Autodesk Inventor part; units mm, degrees
ref_plane "YZ Plane" through (0, 0, 0) normal (1, 0, 0) x (0, 1, 0)
ref_plane "XZ Plane" through (0, 0, 0) normal (0, 1, 0) x (-1, 0, 0)
ref_plane "XY Plane" through (0, 0, 0) normal (0, 0, 1) x (1, 0, 0)
sketch "Skizze1" plane through (0, 0, 0) normal (0, 1, 0) x (-1, 0, 0)
  line L0 (102, -1.5) -> (-102, -1.5)
  line L1 (-102, -1.5) -> (-102, 1.5)
  line L2 (-102, 1.5) -> (102, 1.5)
  line L3 (102, 1.5) -> (102, -1.5)
  line L4 (104, -3.5) -> (-104, -3.5)
  line L5 (-104, -3.5) -> (-104, 3.5)
  line L6 (-104, 3.5) -> (104, 3.5)
  line L7 (104, 3.5) -> (104, -3.5)
  line L8 (0, -4.9) -> (0, 4.9)
  line L9 (-145.6, 0) -> (145.6, 0)
  point P0 (0, 0)
  dimension "d0" = 204
  dimension "d2" = 3
  dimension "d3" = 2
  dimension "d4" = 2
extrude "Extrusion1" add sketch "Skizze1" along normal blind 15 contours L3 L9 L7 L4 L8 L0 | L8 L4 L5 L9 L1 L0 | L3 L2 L8 L6 L7 L9 | L9 L5 L6 L8 L2 L1
sketch "Skizze2" plane through (0, 0, 0) normal (0, 1, 0) x (-1, 0, 0)
  line L0 (104, 3.5) -> (-104, 3.5)
  line L1 (104, -3.5) -> (104, 3.5)
  line L2 (-104, -3.5) -> (104, -3.5)
  line L3 (-104, 3.5) -> (-104, -3.5)
  point P0 (0, 0)
extrude "Extrusion2" add sketch "Skizze2" along normal blind 1
draft "Flächenverjüngung1" angle 10 pull direction (0, 1, 0) faces at (34.6667, 5, -3.5) (104, 10, 1.1667) (-34.6667, 5, 3.5) (-104, 10, -1.1667) fixed edges at (0, 15, -3.5) (104, 15, 0) (0, 15, 3.5) (-104, 15, 0)
properties part number "Stroemungsfilter_Fuss"
Design review of the part built by this model. Coordinates are the model's own, in mm. A direction names the side the tool comes from. Give positions to 0.01 mm unless a question says otherwise; leave off trailing zeros. Write each loop counter-clockwise with the first axis right and the second up, starting at its lowest first coordinate (ties: lowest second). Pieces come first, ordered by that corner, then holes. Notation, with made-up numbers: (77.25, 70) -> (96.25, 70) arc R8 cw to (96.25, 74) -> close; hole circle Ø8 at (4, 51.5). An arc over 180 degrees is marked (long way). Answer in a Markdown table with one row per item.
(1) Consider section A-A (x = 78). State the section outline as (y, z) points.
Results:
| item | result |
|---|---|
| outline | (0, -6.14) -> (15, -3.5) -> (15, -1.5) -> (1, -1.5) -> (1, 1.5) -> (15, 1.5) -> (15, 3.5) -> (0, 6.14) -> close |
(2) For faces 1 (the flat face through (-105.34, 7.39, 0.09)), 2 (the flat face through (1, 8, 1.5)), list the 3-axis set-ups (+Z, -Z, +X, -X, +Y, -Y) from which the entire face can be reached by the end or side of a thin tool; tool diameter is ignored.
Results:
| item | result |
|---|---|
| face 1 | +Z, -Z, -X, +Y |
| face 2 | +Y |
(3) Consider section B-B (y = 6.5). State the section outline as (x, z) points, then the cut area to 3 significant figures.
Results:
| item | result |
|---|---|
| outline | (-105.5, -5) -> (105.5, -5) -> (105.5, 5) -> (-105.5, 5) -> close; hole (-102, -1.5) -> (102, -1.5) -> (102, 1.5) -> (-102, 1.5) -> close |
| area | 1,500 mm2 |
(4) To check wall thickness, follow probe 1 along Z at (x, y) = (92, 11); probe 2 along Z at (x, y) = (32.5, 12.75); probe 3 along X at (y, z) = (9.25, 0.5). State the ranges of each line that lie inside material, in increasing order.
Results:
| item | result |
|---|---|
| probe 1 | -4.21 to -1.5, 1.5 to 4.21 |
| probe 2 | -3.9 to -1.5, 1.5 to 3.9 |
| probe 3 | -105.01 to -102, 102 to 105.01 |
(5) Mouldability with a two-part tool opening along X and no side actions: class faces 3 (the flat face through (-1.49, 7.4, -4.84)), 4 (the flat face through (-1, 8, -1.5)), 5 (the flat face through (105.34, 7.4, -0.09)) as +X half, -X half, draft (parallel to the pull), parting line (faces both ways), or undercut.
Results:
| item | result |
|---|---|
| face 3 | draft |
| face 4 | undercut |
| face 5 | +X half |
(6) Clearance check with flat-ended pins moving along their axes: pin 1 (2.5 mm diameter, centred on y = 8, z = 0.5, fed in from +X); pin 2 (1 mm diameter, centred on x = 3.5, y = 10.5, fed in from +Z); pin 3 (4 mm diameter, centred on y = 11.5, z = -1, fed in from -X). State where each tip first meets the part, or that it passes through.
Results:
| item | result |
|---|---|
| pin 1 | x = 105.45 |
| pin 2 | z = 4.38 |
| pin 3 | x = -104.97 |
